Geometry check sheet. Reference: the model listing, model coordinates, mm. Round coordinates to 2 decimals unless told otherwise and drop trailing zeros. Order: outer loops, then holes, each group sorted by start corner. A loop starts at its lowest first (then second) coordinate and runs counter-clockwise, first axis right, second up. Notation, with made-up numbers: (-7.5, -16.75) -> (6.5, -16.75) arc R33 cw to (6.5, 16.25) -> close; hole circle Ø1 at (47, 14). An arc over 180 degrees is marked (long way). Use a Markdown table: item, result. Add a question column.
Item 1: Sectioned sample at C-C, the plane x = -1.5. Record the cut outline in (y, z).
Item 2: Sectioned sample at A-A, the plane z = 2.75. Record the cut outline in (x, y).
Item 3: Sectioned sample at B-B, the plane y = 7. Record the cut outline in (x, z), and give its area (3 significant figures).
Item 4: Material ranges on probe 1 along Y at (x, z) = (0, 3.25); probe 2 along X at (y, z) = (7.5, 2.5); probe 3 along X at (y, z) = (9.25, 6), recorded low to high. Write a range as [from, to].
Item 5: Gauge pin test, flat ends, axial feed: pin 1 Ø4 at (y, z) = (3, 1) entering from +X; pin 2 Ø1 at (y, z) = (5, 5.5) entering from +X. Record the tip position at first contact, or that the pin passes through.
Item 6: Sectioned sample at D-D, the plane x = -30. Record the cut outline in (y, z).
from build123d import *

# Parameters (mm, degrees)
F1_DEPTH = 7


with BuildPart() as f1:
    # F0 (on Top) → F1 (new body)
    with BuildSketch(Plane.XY):
        with BuildLine():
            ThreePointArc((10.9424882845, 0.9711644524), (10.9747418033, 0.4860582273), (10.9855, 0))
            ThreePointArc((10.9855, 0), (10.9747418033, -0.4860582273), (10.9424882845, -0.9711644524))
            ThreePointArc((10.9424882845, -0.9711644524), (14.7028715464, -8.6649815834), (22.6805508137, -11.7781693116))
            Line((22.6805508137, -11.7781693116), (22.6805508137, -10.9855))
            ThreePointArc((22.6805508137, -10.9855), (11.6950508137, 0), (22.6805508137, 10.9855))
            Line((22.6805508137, 10.9855), (22.6805508137, 11.7781693116))
            ThreePointArc((22.6805508137, 11.7781693116), (14.7028715464, 8.6649815834), (10.9424882845, 0.9711644524))
        make_face()
        with BuildLine():
            ThreePointArc((-10.9423311539, 0.9729332804), (0.0008878968, 10.9854999641), (10.9424882845, 0.9711644524))
            ThreePointArc((10.9424882845, 0.9711644524), (14.7028715464, 8.6649815834), (22.6805508137, 11.7781693116))
            Line((22.6805508137, 11.7781693116), (-22.6802472025, 11.7781693116))
            ThreePointArc((-22.6802472025, 11.7781693116), (-14.7032208322, 8.6655826474), (-10.9423311539, 0.9729332804))
        make_face()
        with BuildLine():
            ThreePointArc((22.6805508137, -11.7781693116), (14.7028715464, -8.6649815834), (10.9424882845, -0.9711644524))
            ThreePointArc((10.9424882845, -0.9711644524), (0.0008878968, -10.9854999641), (-10.9423311539, -0.9729332804))
            ThreePointArc((-10.9423311539, -0.9729332804), (-14.7032208322, -8.6655826474), (-22.6802472025, -11.7781693116))
            Line((-22.6802472025, -11.7781693116), (22.6805508137, -11.7781693116))
        make_face()
        with BuildLine():
            ThreePointArc((-10.9423311539, -0.9729332804), (-10.9855, 0), (-10.9423311539, 0.9729332804))
            ThreePointArc((-10.9423311539, 0.9729332804), (-14.7032208322, 8.6655826474), (-22.6802472025, 11.7781693116))
            Line((-22.6802472025, 11.7781693116), (-22.6802472025, 10.9855))
            ThreePointArc((-22.6802472025, 10.9855), (-14.9123256578, 7.7679215447), (-11.6947472025, 0))
            ThreePointArc((-11.6947472025, 0), (-14.9123256578, -7.7679215447), (-22.6802472025, -10.9855))
            Line((-22.6802472025, -10.9855), (-22.6802472025, -11.7781693116))
            ThreePointArc((-22.6802472025, -11.7781693116), (-14.7032208322, -8.6655826474), (-10.9423311539, -0.9729332804))
        make_face()
        with BuildLine():
            ThreePointArc((34.4587201253, 0), (31.0089742039, 8.3284233902), (22.6805508137, 11.7781693116))
            Line((22.6805508137, 11.7781693116), (22.6805508137, 10.9855))
            ThreePointArc((22.6805508137, 10.9855), (30.4484723584, 7.7679215447), (33.6660508137, 0))
            ThreePointArc((33.6660508137, 0), (30.4484723584, -7.7679215447), (22.6805508137, -10.9855))
            Line((22.6805508137, -10.9855), (22.6805508137, -11.7781693116))
            ThreePointArc((22.6805508137, -11.7781693116), (31.0089742039, -8.3284233902), (34.4587201253, 0))
        make_face()
        with BuildLine():
            Line((-22.6802472025, 10.9855), (-22.6802472025, 11.7781693116))
            ThreePointArc((-22.6802472025, 11.7781693116), (-34.4584165141, 0), (-22.6802472025, -11.7781693116))
            Line((-22.6802472025, -11.7781693116), (-22.6802472025, -10.9855))
            ThreePointArc((-22.6802472025, -10.9855), (-33.6657472025, 0), (-22.6802472025, 10.9855))
        make_face()
        with BuildLine():
            Line((-22.6802472025, -10.9855), (-22.6802472025, 10.9855))
            ThreePointArc((-22.6802472025, 10.9855), (-33.6657472025, 0), (-22.6802472025, -10.9855))
        make_face()
        with BuildLine():
            ThreePointArc((-11.6947472025, 0), (-14.9123256578, 7.7679215447), (-22.6802472025, 10.9855))
            Line((-22.6802472025, 10.9855), (-22.6802472025, -10.9855))
            ThreePointArc((-22.6802472025, -10.9855), (-14.9123256578, -7.7679215447), (-11.6947472025, 0))
        make_face()
        with BuildLine():
            Line((22.6805508137, -10.9855), (22.6805508137, 10.9855))
            ThreePointArc((22.6805508137, 10.9855), (11.6950508137, 0), (22.6805508137, -10.9855))
        make_face()
        with BuildLine():
            ThreePointArc((33.6660508137, 0), (30.4484723584, 7.7679215447), (22.6805508137, 10.9855))
            Line((22.6805508137, 10.9855), (22.6805508137, -10.9855))
            ThreePointArc((22.6805508137, -10.9855), (30.4484723584, -7.7679215447), (33.6660508137, 0))
        make_face()
    extrude(amount=F1_DEPTH)


solid = f1.part
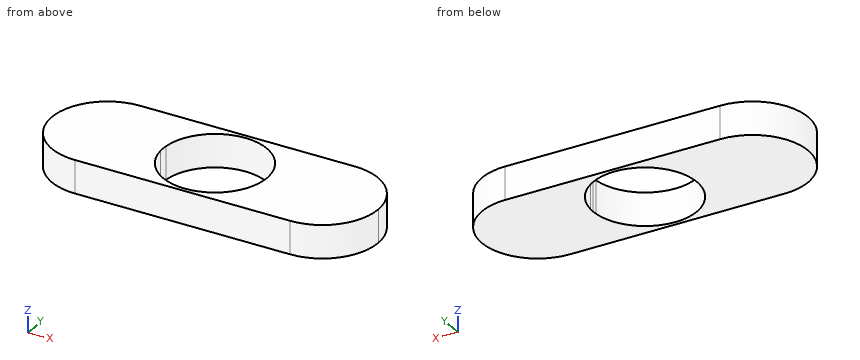
Found:
| question | item | result |
|---|---|---|
| 1 | outline | (-11.78, 0) -> (-10.88, 0) -> (-10.88, 7) -> (-11.78, 7) -> close; (10.88, 0) -> (11.78, 0) -> (11.78, 7) -> (10.88, 7) -> close |
| 2 | outline | (-22.68, -11.78) -> (22.68, -11.78) arc R11.78 ccw to (22.68, 11.78) -> (-22.68, 11.78) arc R11.78 ccw to start; hole circle Ø21.97 at (0, 0) |
| 3 | outline | (-32.15, 0) -> (-8.47, 0) -> (-8.47, 7) -> (-32.15, 7) -> close; (8.47, 0) -> (32.15, 0) -> (32.15, 7) -> (8.47, 7) -> close |
| 3 | area | 332 mm2 |
| 4 | probe 1 | y = [-11.78, -10.99], [10.99, 11.78] |
| 4 | probe 2 | x = [-31.76, -8.03], [8.03, 31.76] |
| 4 | probe 3 | x = [-29.97, -5.93], [5.93, 29.97] |
| 5 | pin 1 | stops at x = 34.42 |
| 5 | pin 2 | stops at x = 33.57 |
| 6 | outline | (-9.23, 0) -> (9.23, 0) -> (9.23, 7) -> (-9.23, 7) -> close |
